from build123d import *

# Parameters (mm, degrees)
F0_W     = 88
F0_H     = 88
F1_DEPTH = 720
F2_W     = 30
F2_H     = 29
F3_DEPTH = 88.001
F4_W     = 30
F4_H     = 29
F5_DEPTH = 88.001
F6_R     = 5


with BuildPart() as f1:
    # F0 (on Right) → F1 (new body)
    with BuildSketch(Plane.YZ):
        with Locations((44, 44)):
            Rectangle(F0_W, F0_H)
    extrude(amount=F1_DEPTH)

    # F2 (on face) → F3 (cut, through all)
    with BuildSketch(Plane.XY.offset(88)):
        with Locations((705, 14.5)):
            Rectangle(F2_W, F2_H)
        with Locations((705, 73.5)):
            Rectangle(F2_W, F2_H)
    extrude(amount=-F3_DEPTH, mode=Mode.SUBTRACT)

    # F4 (on face) → F5 (cut, through all)
    with BuildSketch(Plane.XY.offset(88)):
        with Locations((15, 73.5)):
            Rectangle(F4_W, F4_H)
        with Locations((15, 14.5)):
            Rectangle(F4_W, F4_H)
    extrude(amount=-F5_DEPTH, mode=Mode.SUBTRACT)

    # F6
    f6_edges = [f1.edges().sort_by_distance(p)[0] for p in [
        (30, 0, 44),
        (360, 0, 0),
        (690, 0, 44),
        (360, 0, 88),
        (360, 88, 88),
        (360, 88, 0),
        (690, 88, 44),
        (30, 88, 44),
    ]]
    fillet(f6_edges, radius=F6_R)


solid = f1.part
Check sheet for the modelled part. Datum: model origin and axes. Units: mm. A direction names the side the tool comes from. Give positions to 0.01 mm unless a question says otherwise; leave off trailing zeros. Write each loop counter-clockwise with the first axis right and the second up, starting at its lowest first coordinate (ties: lowest second). Pieces come first, ordered by that corner, then holes. Notation, with made-up numbers: (60, 66) -> (103, 66) arc R24 ccw to (103, 91) -> close; hole circle Ø6 at (73, 53). An arc over 180 degrees is marked (long way). Use one line per item in the form item = value. Start each with the question number.
1. Access from +Z, -Z, +X, -X, +Y, -Y to the whole of each face (thin tool, end or side, straight path). Record for faces 1 (the flat face through (705, 59, 45)), 2 (the flat face through (355, 0, 43)), 3 (the flat face through (15, 29, 45)), 4 (the flat face through (30, 71, 45)), 5 (the flat face through (690, 17, 45)).
2. Section check A-A (z = 15.5). Record the cut outline in (x, y), and give its area (3 significant figures).
3. Section check B-B (y = 68.5). Record the cut outline in (x, z), and give its area (3 significant figures).
4. Thickness scan on line 1 along X through (y, z) = (67, 38.5); line 2 along Y through (x, z) = (549, 4.5); line 3 along X through (y, z) = (4, 67). Record the ranges inside material, lowest first. Write a range as from..to.
5. Go/stop test with flat-tipped pins: P1, Ø24, axis at x = 708, z = 56, coming from the -Y side; P2, Ø7, axis at y = 73, z = 53.5, coming from the +X side; P3, Ø12, axis at y = 16.5, z = 61, coming from the -X side. Record where each tip stops, or that it passes through.
Conclusion:
q1.face_1 = +Z, -Z, +X, +Y
q1.face_2 = +Z, -Z, +X, -X, -Y
q1.face_3 = +Z, -Z, -X, -Y
q1.face_4 = +Z, -Z, -X, +Y
q1.face_5 = +Z, -Z, +X, -Y
q2.outline = (0, 29) -> (30, 29) -> (30, 5) arc R5 ccw to (35, 0) -> (685, 0) arc R5 ccw to (690, 5) -> (690, 29) -> (720, 29) -> (720, 59) -> (690, 59) -> (690, 83) arc R5 ccw to (685, 88) -> (35, 88) arc R5 ccw to (30, 83) -> (30, 59) -> (0, 59) -> close
q2.area = 59,900 mm²
q3.outline = (30, 0) -> (690, 0) -> (690, 88) -> (30, 88) -> close
q3.area = 58,100 mm²
q4.line_1 = 30..690
q4.line_2 = 0.03..87.97
q4.line_3 = 30.1..689.9
q5.P1 = 29
q5.P2 = 690
q5.P3 = 30
